```python
from build123d import *

# Parameters (mm, degrees)
Y_KSEKLIK_EKSTR_ZYON1_DEPTH = 310


with BuildPart() as part:
    # Çizim1 → Yükseklik-Ekstrüzyon1 (new body)
    with BuildSketch(Plane(origin=(0, 0, 0), x_dir=(0, -1, 0), z_dir=(-1, 0, 0))):
        Polygon((0, 0), (-4, 0), (-4, -4), (-3.5, -4), (-3.5, -0.5), (-0.5, -0.5), (-0.5, -13.15), (-3.5, -13.15), (-3.5, -9.65), (-4, -9.65), (-4, -13.65), (0, -13.65), align=None)
    extrude(amount=-Y_KSEKLIK_EKSTR_ZYON1_DEPTH)


solid = part.part
```
Read the model definition and answer for the solid it produces. Units are mm, in the model's axes. Give positions to 0.01 mm unless a question says otherwise; leave off trailing zeros. Write each loop counter-clockwise with the first axis right and the second up, starting at its lowest first coordinate (ties: lowest second). Pieces come first, ordered by that corner, then holes. Notation, with made-up numbers: (87.25, 83.5) - (103.25, 83.5) arc R22 cw to (103.25, 104.5) - close; hole circle Ø3 at (84, 12.5). An arc over 180 degrees is marked (long way). Write item = value, one per line. Start each with the question number.
Item 1: Each of these flat-tipped pins is pushed along its axis until it touches: P1, Ø0.6, axis at x = 163, y = 3.5, coming from the +Z side; P2, Ø2, axis at y = 2, z = -4, coming from the -X side. Where does it stop, or does it pass through?
Item 2: Find the intervals of material crossed by probe 1 along Y at (x, z) = (165.5, -1.5); probe 2 along Z at (x, y) = (269, 2.35); probe 3 along Z at (x, y) = (49.5, 3.65), in increasing order. Write a range as [from, to].
Item 3: Find section C-C (z = -6.25). Give the vertices of the cut face in (x, y).
Item 4: The mould has two halves that part along Y. Classify faces 1 (the flat face through (153, 0.5, -7)), 2 (the flat face through (153, 0, -7)): +Y half, -Y half, draft (parallel to the pull), parting line (faces both ways), or undercut.
Item 5: Find section A-A (y = 2.45). Give the vertices of the cut face in (x, z), then the cut area to 3 significant figures.
Item 6: Find section B-B (x = 289). Give the vertices of the cut face in (y, z), then the cut area to 3 significant figures.
Response:
q1.P1 = 0
q1.P2 = through
q2.probe_1 = [0, 0.5], [3.5, 4]
q2.probe_2 = [-13.65, -13.15], [-0.5, 0]
q2.probe_3 = [-13.65, -9.65], [-4, 0]
q3.outline = (0, 0) - (310, 0) - (310, 0.5) - (0, 0.5) - close
q4.face_1 = undercut
q4.face_2 = -Y half
q5.outline = (0, -13.65) - (310, -13.65) - (310, -13.15) - (0, -13.15) - close; (0, -0.5) - (310, -0.5) - (310, 0) - (0, 0) - close
q5.area = 310 mm²
q6.outline = (0, -13.65) - (4, -13.65) - (4, -9.65) - (3.5, -9.65) - (3.5, -13.15) - (0.5, -13.15) - (0.5, -0.5) - (3.5, -0.5) - (3.5, -4) - (4, -4) - (4, 0) - (0, 0) - close
q6.area = 13.8 mm²
